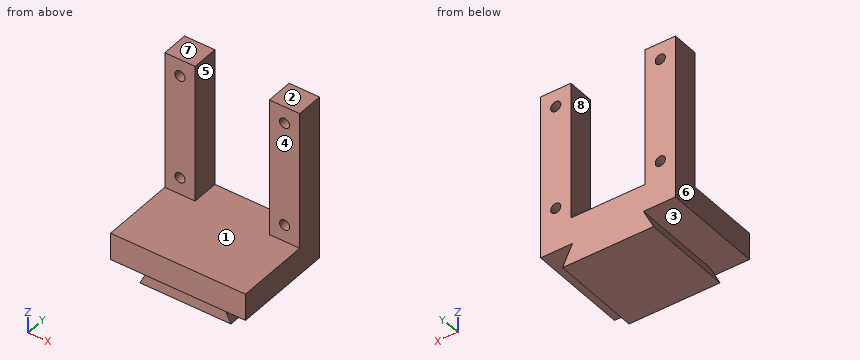
from build123d import *

# Parameters (mm, degrees)
F1_DEPTH = 27
F2_R     = 1.5
F3_DEPTH = 8
F4_W     = 40
F4_H     = 8
F5_DEPTH = 30


with BuildPart() as f1:
    # F0 (on Front) → F1 (new body)
    with BuildSketch(Plane.XZ):
        Polygon((-10.5, 6), (-13.5, 0), (13.5, 0), (10.5, 6), align=None)
    extrude(amount=F1_DEPTH)

    # F2 (on Front) → F3 (join)
    with BuildSketch(Plane.XZ):
        Polygon((-10.5, 6), (10.5, 6), (20, 6), (20, 55), (11, 55), (11, 14), (-11, 14), (-11, 55), (-20, 55), (-20, 6), align=None)
        with Locations((-15.5, 19)):
            Circle(F2_R, mode=Mode.SUBTRACT)
        with Locations((15.5, 19)):
            Circle(F2_R, mode=Mode.SUBTRACT)
        with Locations((-15.5, 50)):
            Circle(F2_R, mode=Mode.SUBTRACT)
        with Locations((15.5, 50)):
            Circle(F2_R, mode=Mode.SUBTRACT)
    extrude(amount=F3_DEPTH)

    # F4 (on Front) → F5 (join)
    with BuildSketch(Plane.XZ):
        with Locations((0, 10)):
            Rectangle(F4_W, F4_H)
    extrude(amount=F5_DEPTH)


solid = f1.part
Can you work these out from the model? Positions are in its coordinate system, mm. Face numbers are marked on the shaded views. A direction names the side the tool comes from. Coordinates: 2 decimals unless noted, no trailing zeros. Loops run counter-clockwise (first coordinate to the right, second up) from the corner with the lowest first, then second, coordinate; pieces in that order, holes last. Notation, with made-up numbers: (64.5, -18) - (101.5, -18) arc R15 ccw to (101.5, 5) - close; hole circle Ø3 at (71.25, -12). An arc over 180 degrees is marked (long way). Answer as a JSON object with one key per item and string values. Group by question number.
Item 1: If I drill on L1, parallel to Z at x = -15.5, y = -6; L2, parallel to X at y = -2.75, z = 37.5; L3, parallel to Z at x = 3, y = -14, over which ranges is the centre line in solid material (lowest first)? Write a range as from..to.
Item 2: If we section it at A-A (x = 15.5): List the corners of the cut face in (y, z) for me, plus the area to 3 significant figures.
Item 3: If we mould it in two halves opening along X, with no side actions, what happens to the marked faces 6, 7 and 8? For each: released by +X, released by -X, zero draft, split by the parting line, or undercut.
Item 4: If we section it at C-C (y = -6): List the corners of the cut face in (x, z) for me.
Item 5: If we section it at B-B (z = 29.5): List the corners of the cut face in (x, y) for me, plus the area to 3 significant figures.
Item 6: If we section it at D-D (z = 50): List the corners of the cut face in (x, y) for me.
Item 7: On a 3-axis mill with a long thin cutter (end or side, diameter ignored), from which of +Z, -Z, +X, -X, +Y, -Y can I reach the whole of each face in a straight line? I mean the marked faces 1, 2, 3, 4 and 5. Say none if no direction works.
Item 8: For pin 1 (4 mm diameter, centred on x = 15.5, z = 50, fed in from -Y); pin 2 (3 mm diameter, centred on x = -2, z = 4, fed in from -Y), each with a flat end and sliding along its axis, tell me the tip position at first contact or that it passes through.
Returned:
{
 "1": {"L1": "z = 6..17.5, 20.5..48.5, 51.5..55", "L2": "x = -20..-11, 11..20", "L3": "z = 0..14"},
 "2": {"outline": "(-30, 6) - (0, 6) - (0, 17.5) - (-8, 17.5) - (-8, 14) - (-30, 14) - close; (-8, 20.5) - (0, 20.5) - (0, 48.5) - (-8, 48.5) - close; (-8, 51.5) - (0, 51.5) - (0, 55) - (-8, 55) - close", "area": "520 mm²"},
 "3": {"face 6": "released by -X", "face 7": "zero draft", "face 8": "undercut"},
 "4": {"outline": "(-20, 6) - (-10.5, 6) - (-13.5, 0) - (13.5, 0) - (10.5, 6) - (20, 6) - (20, 55) - (11, 55) - (11, 14) - (-11, 14) - (-11, 55) - (-20, 55) - close; hole circle Ø3 at (-15.5, 19); hole circle Ø3 at (-15.5, 50); hole circle Ø3 at (15.5, 19); hole circle Ø3 at (15.5, 50)"},
 "5": {"outline": "(-20, -8) - (-11, -8) - (-11, 0) - (-20, 0) - close; (11, -8) - (20, -8) - (20, 0) - (11, 0) - close", "area": "144 mm²"},
 "6": {"outline": "(-20, -8) - (-17, -8) - (-17, 0) - (-20, 0) - close; (-14, -8) - (-11, -8) - (-11, 0) - (-14, 0) - close; (11, -8) - (14, -8) - (14, 0) - (11, 0) - close; (17, -8) - (20, -8) - (20, 0) - (17, 0) - close"},
 "7": {"face 1": "+Z, -Y", "face 2": "+Z, +X, -X, +Y, -Y", "face 3": "-Y", "face 4": "+Z, +X, -X, -Y", "face 5": "+Z, +Y, -Y"},
 "8": {"pin 1": "stops at y = -8", "pin 2": "stops at y = -27"}
}
